The figure shows three views and two pictorial views of one solid part (mm, origin at its lowest corner). Answer the questions. Coordinates: 2 decimals unless noted, no trailing zeros. Order: outer loops, then holes, each group sorted by start corner. A loop starts at its lowest first (then second) coordinate and runs counter-clockwise, first axis right, second up. Notation, with made-up numbers: (1, -14.5) - (60, -14.5) arc R6 cw to (60, -8.5) - close; hole circle Ø7 at (84, 44). An arc over 180 degrees is marked (long way). Use one line per item in the form item = value. Start each with the question number.
Item 1: This flat-tipped pin is pushed along its axis until it touches: pin 1 Ø3 at (x, z) = (86, 6) entering from +Y. Where does it stop, or does it pass through?
Item 2: Section B-B, the plane y = 1.1 is taken. Write down the section's boundary in (x, z).
Item 3: Section A-A, the plane x = 237.5 is taken. Write down the section's boundary in (y, z), and give its area (3 significant figures).
Item 4: Consider line 1 along X through (y, z) = (1.2, 14.25); line 2 along Z through (x, y) = (71, 1.15); line 3 along Z through (x, y) = (237.5, 1.05). Determine where each line is inside the solid, lowest interval first. Write a range as [from, to].
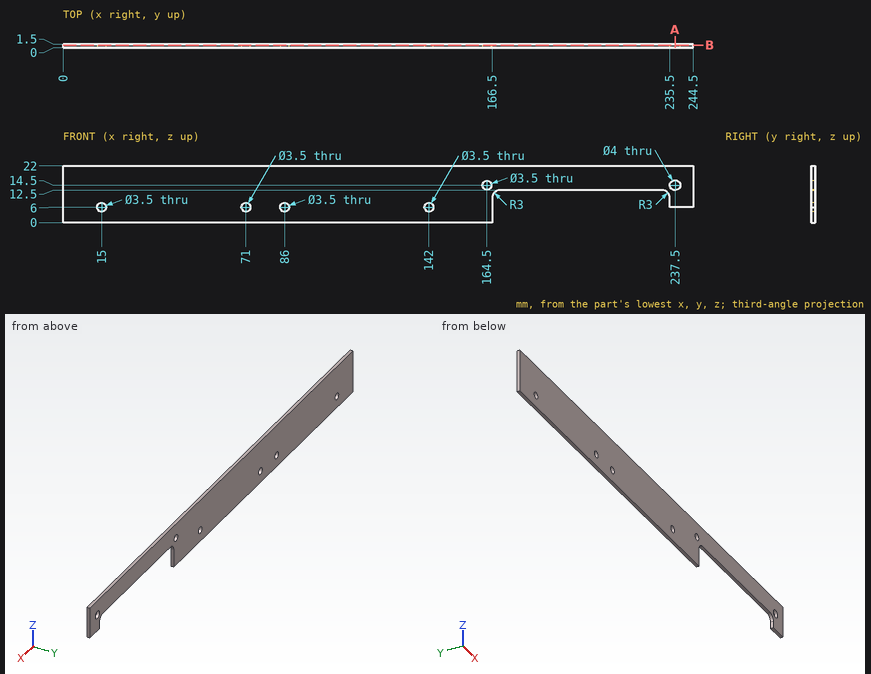
Response:
q1.pin_1 = through
q2.outline = (0, 0) - (166.5, 0) - (166.5, 9.5) arc R3 cw to (169.5, 12.5) - (232.5, 12.5) arc R3 cw to (235.5, 9.5) - (235.5, 6) - (244.5, 6) - (244.5, 22) - (0, 22) - close; hole circle Ø3.5 at (15, 6); hole circle Ø3.5 at (71, 6); hole circle Ø3.5 at (86, 6); hole circle Ø3.5 at (142, 6); hole circle Ø3.5 at (164.5, 14.5); hole circle Ø4 at (237.5, 14.5)
q3.outline = (0, 6) - (1.5, 6) - (1.5, 12.5) - (0, 12.5) - close; (0, 16.5) - (1.5, 16.5) - (1.5, 22) - (0, 22) - close
q3.area = 18.0 mm2
q4.line_1 = [0, 162.77], [166.23, 235.52], [239.48, 244.5]
q4.line_2 = [0, 4.25], [7.75, 22]
q4.line_3 = [6, 12.5], [16.5, 22]
